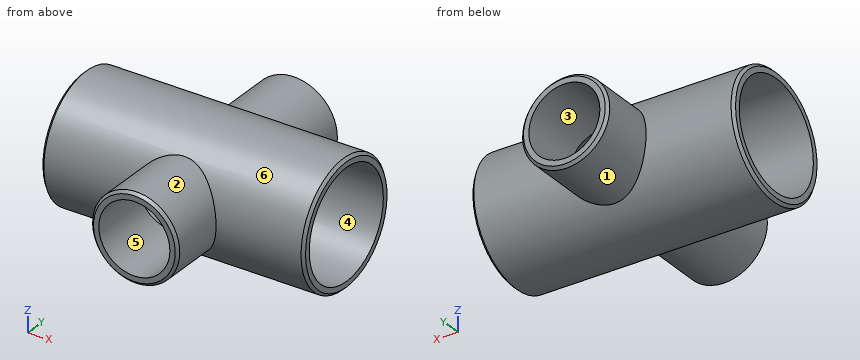
from build123d import *

# Parameters (mm, degrees)
RUNROUTE_R          = 30.1625
RUNEXTRUDE_DEPTH    = 63.5
OUTLETROUTE_R       = 21.082
OUTLETEXTRUDE_DEPTH = 57.15
CROSSSHELL_T        = -3.9116
CROSSCHAMFER_SIZE   = 1.303866667


with BuildPart() as part:
    # RunRoute → RunExtrude (new body)
    with BuildSketch(Plane(origin=(0, 0, 0), x_dir=(0, 0, -1), z_dir=(1, 0, 0))):
        Circle(RUNROUTE_R)
    runextrude = extrude(amount=RUNEXTRUDE_DEPTH)

    # RunExtrudeMirror: RunExtrude across plane
    add(runextrude.mirror(Plane(origin=(0, 0, 0), x_dir=(0, 0, 1), z_dir=(1, 0, 0))))

    # OutletRoute → OutletExtrude (add)
    with BuildSketch(Plane(origin=(0, 0, 0), x_dir=(1, 0, 0), z_dir=(0, 1, 0))):
        with Locations(Location((0, 0, 0), (0, 0, 90))):
            Circle(OUTLETROUTE_R)
    outletextrude = extrude(amount=OUTLETEXTRUDE_DEPTH)

    # OutletExtrudeMirror: OutletExtrude across plane
    add(outletextrude.mirror(Plane.ZX))

    # CrossShell
    crossshell_openings = [part.faces().sort_by_distance(p)[0] for p in [
        (63.5, 0, 0),
        (0, 57.15, 0),
        (0, -57.15, 0),
        (-63.5, 0, 0),
    ]]
    offset(amount=CROSSSHELL_T, openings=crossshell_openings, kind=Kind.INTERSECTION)

    # CrossChamfer
    crosschamfer_edges = [part.edges().sort_by_distance(p)[0] for p in [
        (0, -57.15, 21.082),
        (63.5, 0, 30.1625),
        (-63.5, 0, 30.1625),
        (0, 57.15, 21.082),
    ]]
    chamfer(crosschamfer_edges, length=CROSSCHAMFER_SIZE)


solid = part.part
Source: CAD feature listing. Evaluate the final solid. Frame: model axes, mm. Face numbers are marked on the shaded views. A direction names the side the tool comes from. Give positions to 0.01 mm unless a question says otherwise; leave off trailing zeros. Write each loop counter-clockwise with the first axis right and the second up, starting at its lowest first coordinate (ties: lowest second). Pieces come first, ordered by that corner, then holes. Notation, with made-up numbers: (41, 18.5) - (67, 18.5) arc R30 cw to (67, 41.5) - close; hole circle Ø6 at (-2, 38). An arc over 180 degrees is marked (long way). Write item = value, one per line. Start each with the question number.
Q1. Cut plane C-C, the plane y = 49. Return loops of the section in (x, z).
Q2. Draft query along Z for the marked faces 4, 5 and 6. Return one class per face: +Z half, -Z half, draft (parallel to the pull), parting line (faces both ways), or undercut.
Q3. Cut plane D-D, the plane x = 24.5. Return loops of the section in (y, z) (1 decimal), then the cut area to 3 significant figures.
Q4. Reachability of the marked faces 1, 2 and 3 from +Z, -Z, +X, -X, +Y, -Y: full face, straight path, thin tool, end or side. Return the list, or none.
Q5. Material intervals for probe 1 along Y at (x, z) = (24, 0); probe 2 along X at (y, z) = (-43, -1); probe 3 along Y at (x, z) = (-45.5, 6.5), sorted ascending.
Q6. Pin query (flat end, axial travel): pin 1 Ø10 at (x, z) = (-49.5, -3.5) entering from +Y; pin 2 Ø2 at (x, z) = (24, 18.5) entering from -Y; pin 3 Ø3 at (y, z) = (-32, 13.5) entering from -X; pin 4 Ø2 at (x, z) = (-7, -14.5) entering from +Y. Return the tip coordinate at first contact, or that it passes through.
Q7. Cut plane A-A, the plane z = 0. Give the number of separate pieces and of enclosed holes in the cut face, then the cut area to 3 significant figures.
Q8. Cut plane B-B, the plane y = 0. Return loops of the section in (x, z), then the cut area to 3 significant figures.
Computed values:
q1.outline = circle Ø42.16 at (0, 0); hole circle Ø34.34 at (0, 0)
q2.face_4 = undercut
q2.face_5 = undercut
q2.face_6 = parting line
q3.outline = circle Ø60.3 at (0, 0); hole circle Ø52.5 at (0, 0)
q3.area = 693 mm²
q4.face_1 = +Y
q4.face_2 = -Y
q4.face_3 = +Y, -Y
q5.probe_1 = -30.16 to -26.25, 26.25 to 30.16
q5.probe_2 = -21.06 to -17.14, 17.14 to 21.06
q5.probe_3 = -29.45 to -25.43, 25.43 to 29.45
q6.pin_1 = 30.16
q6.pin_2 = -24.57
q6.pin_3 = -17.33
q6.pin_4 = through
q7.separate_pieces = 4
q7.enclosed_holes = 0
q7.area = 1,140 mm²
q8.outline = (-63.5, -28.86) - (-62.2, -30.16) - (62.2, -30.16) - (63.5, -28.86) - (63.5, -26.25) - (-63.5, -26.25) - close; (-63.5, 26.25) - (63.5, 26.25) - (63.5, 28.86) - (62.2, 30.16) - (-62.2, 30.16) - (-63.5, 28.86) - close
q8.area = 990 mm²
